Part model, mm, in its own coordinate system. Face numbers are marked on the shaded views. Coordinates: 2 decimals unless noted, no trailing zeros. Write each loop counter-clockwise with the first axis right and the second up, starting at its lowest first coordinate (ties: lowest second). Pieces come first, ordered by that corner, then holes. Notation, with made-up numbers: M -20.75,3 L -15.75,3 A16 ccw -15.75,28 Z; hole C 61,-3.75 d3. An arc over 180 degrees is marked long. Use a Markdown table: item, result. Add a question column.
Q1. Slice it at C-C on z = 65. Write the cut outline in (x, y), then the cut area to 3 significant figures.
Q2. Mould opens along Y. For the marked faces 1 and 2 say: released by +Y, released by -Y, zero draft, split by the parting line, or undercut.
Q3. Wall check: L1, parallel to X at y = 0, z = 63; L2, parallel to Y at x = 0, z = 155; L3, parallel to X at y = 0, z = 154.5. Give the ranges that are in metal, low to high. Write a range as from..to.
Q4. Slice it at A-A on y = 0. Write the cut outline in (x, z), then the cut area to 3 significant figures.
Q5. Slice it at D-D on y = 16. Write the cut outline in (x, z).
Q6. Pin check, flat tips, straight feed: pin 1 Ø6 at (x, z) = (-17.5, 96.5) entering from +Y; pin 2 Ø1.5 at (x, z) = (-5.5, 37) entering from -Y; pin 3 Ø3 at (x, z) = (7.5, 134.5) entering from +Y; pin 4 Ø12 at (x, y) = (0, 0) entering from -Z. Stop position of each tip, or through.
Q7. Slice it at B-B on x = 0. Write the cut outline in (y, z), then the cut area to 3 significant figures.
from build123d import *

# Parameters (mm, degrees)
BOSS_EXTRUDE1_DEPTH = 152.4
SKETCH3_R           = 21
BOSS_EXTRUDE2_DEPTH = 7
BOSS_EXTRUDE3_START = -152.4
BOSS_EXTRUDE3_DEPTH = 152.4


with BuildPart() as part:
    # Sketch1 → Boss-Extrude1 (new body)
    with BuildSketch(Plane.XY):
        with BuildLine():
            Line((-2.5, 22.25), (-2.5, 24.874685928))
            ThreePointArc((-2.5, 24.874685928), (-25, 0), (-2.5, -24.874685928))
            Line((-2.5, -24.874685928), (-2.5, -9.682458366))
            ThreePointArc((-2.5, -9.682458366), (0, 10), (2.5, -9.682458366))
            Line((2.5, -9.682458366), (2.5, -24.874685928))
            ThreePointArc((2.5, -24.874685928), (25, 0), (2.5, 24.874685928))
            Line((2.5, 24.874685928), (2.5, 22.25))
            Line((2.5, 22.25), (-2.5, 22.25))
        make_face()
    extrude(amount=BOSS_EXTRUDE1_DEPTH)

    # Sketch3 → Boss-Extrude2 (add)
    with BuildSketch(Plane.XY.offset(152.4)):
        with BuildLine():
            Line((-2.5, 22.25), (2.5, 22.25))
            Line((2.5, 22.25), (2.5, 24.874685928))
            ThreePointArc((2.5, 24.874685928), (24.874685928, -2.5), (-2.5, -24.874685928))
            ThreePointArc((-2.5, -24.874685928), (-25, 0), (-2.5, 24.874685928))
            Line((-2.5, 24.874685928), (-2.5, 22.25))
        make_face()
        with Locations(Location((0, 0, 0), (0, 0, 263.162858832))):
            Circle(SKETCH3_R, mode=Mode.SUBTRACT)
    extrude(amount=BOSS_EXTRUDE2_DEPTH)

    # Sketch4 → Boss-Extrude3 (add)
    with BuildSketch(Plane.XY.offset(152.4).offset(BOSS_EXTRUDE3_START)):
        with BuildLine():
            Line((-2.5, -14.790199458), (-2.5, -24.874685928))
            ThreePointArc((-2.5, -24.874685928), (0, -25), (2.5, -24.874685928))
            Line((2.5, -24.874685928), (2.5, -14.790199458))
            ThreePointArc((2.5, -14.790199458), (0, -15), (-2.5, -14.790199458))
        make_face()
    extrude(amount=BOSS_EXTRUDE3_DEPTH)


solid = part.part
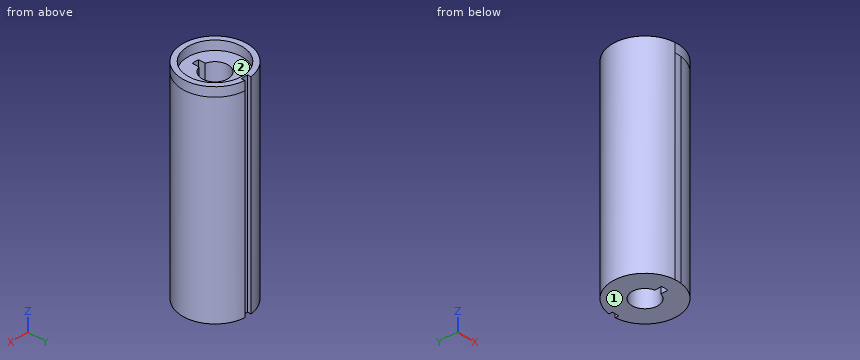
Recorded:
| question | item | result |
|---|---|---|
| 1 | outline | M -2.5,22.25 L -2.5,24.87 A25 ccw long 2.5,24.87 L 2.5,22.25 Z; hole M -2.5,-14.79 A15 ccw 2.5,-14.79 L 2.5,-9.68 A10 ccw long -2.5,-9.68 Z |
| 1 | area | 1,610 mm² |
| 2 | face 1 | zero draft |
| 2 | face 2 | undercut |
| 3 | L1 | -25..-10, 10..25 |
| 3 | L2 | -25..-21, 21..22.25 |
| 3 | L3 | -25..-21, 21..25 |
| 4 | outline | M -25,0 L -10,0 L -10,152.4 L -21,152.4 L -21,159.4 L -25,159.4 Z; M 10,0 L 25,0 L 25,159.4 L 21,159.4 L 21,152.4 L 10,152.4 Z |
| 4 | area | 4,630 mm² |
| 5 | outline | M -19.21,0 L 19.21,0 L 19.21,159.4 L 13.6,159.4 L 13.6,152.4 L -13.6,152.4 L -13.6,159.4 L -19.21,159.4 Z |
| 6 | pin 1 | y = 20.37 |
| 6 | pin 2 | y = -24.54 |
| 6 | pin 3 | y = 24.27 |
| 6 | pin 4 | through |
| 7 | outline | M -25,0 L -15,0 L -15,152.4 L -21,152.4 L -21,159.4 L -25,159.4 Z; M 10,0 L 22.25,0 L 22.25,159.4 L 21,159.4 L 21,152.4 L 10,152.4 Z |
| 7 | area | 3,430 mm² |
